The figure shows three views and two pictorial views of one solid part (mm, origin at its lowest corner). Answer the questions. Coordinates: 2 decimals unless noted, no trailing zeros. Order: outer loops, then holes, each group sorted by start corner. A loop starts at its lowest first (then second) coordinate and runs counter-clockwise, first axis right, second up. Notation, with made-up numbers: M 55.25,71 L 76.25,71 A7 cw 76.25,82 Z; hole C -36,64.5 d6. An arc over 180 degrees is marked long. Answer in a Markdown table with one row per item. Add a question column.
Item 1: The mould has two halves that part along X. Classify the marked faces 1, 2 and 3: released by +X, released by -X, zero draft, split by the parting line, or undercut.
Item 2: The part is cut by section C-C (z = 33.5). Write down the section's boundary in (x, y).
Item 3: The part is cut by section A-A (y = 2). State how many separate pieces and enclosed holes the cut face has.
Item 4: Flat-ended cylindrical pins translate along their axes: pin 1 Ø3 at (x, z) = (10.38, 29.63) entering from -Y; pin 2 Ø2 at (y, z) = (2, 22) entering from -X; pin 3 Ø1.7 at (x, z) = (2.69, 18.73) entering from +Y. Find the tip coordinate at first contact, or state that the pin passes through.
Item 5: Consider line 1 (X direction, y = 2, z = 18) (1 decimal); line 2 (X direction, y = 0.5, z = 18.5) (1 decimal); line 3 (X direction, y = 4.25, z = 11) (1 decimal). Determine where each line is inside the solid, lowest interval first. Write a range as from..to.
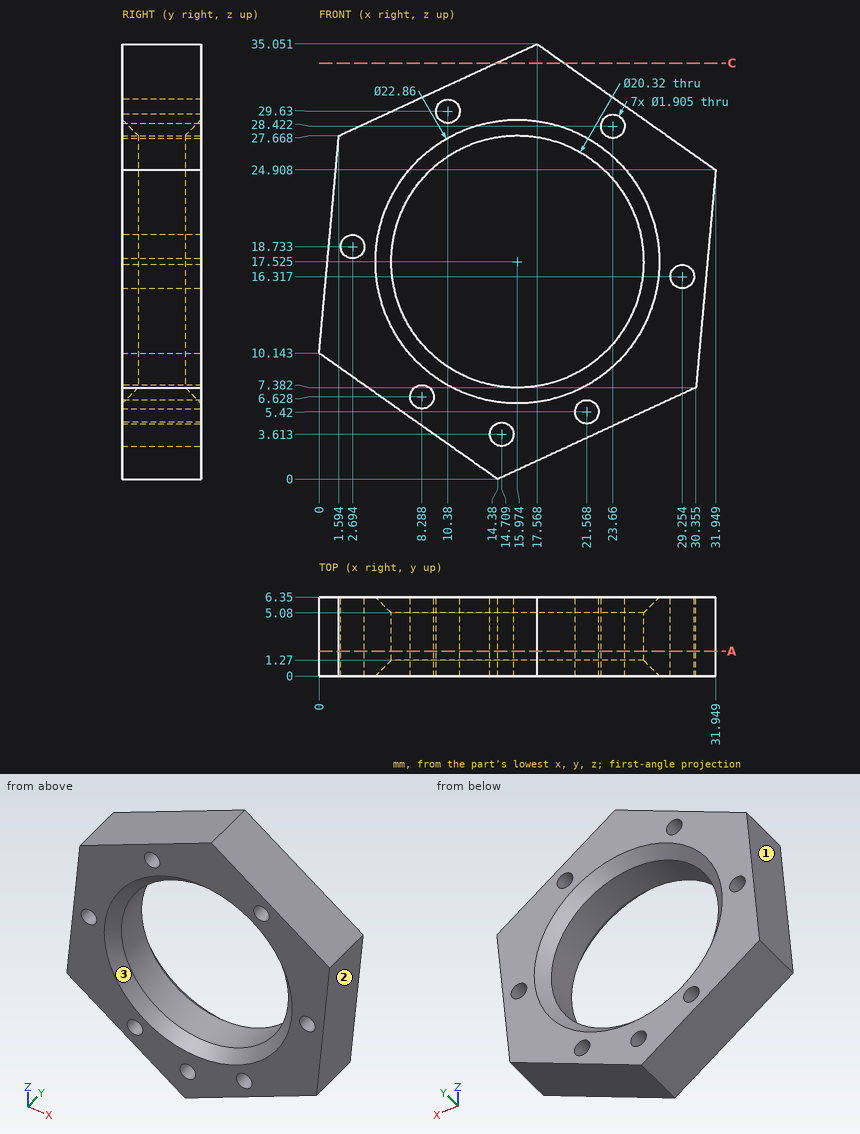
Reply:
| question | item | result |
|---|---|---|
| 1 | face 1 | released by -X |
| 1 | face 2 | released by +X |
| 1 | face 3 | undercut |
| 2 | outline | M 14.21,0 L 19.77,0 L 19.77,6.35 L 14.21,6.35 Z |
| 3 | separate pieces | 1 |
| 3 | enclosed holes | 8 |
| 4 | pin 1 | stops at y = 0 |
| 4 | pin 2 | stops at x = 0.99 |
| 4 | pin 3 | passes through |
| 5 | line 1 | x = 0.7..2.1, 3.3..5.8, 26.1..31.3 |
| 5 | line 2 | x = 0.8..1.8, 3.6..5.1, 26.9..31.4 |
| 5 | line 3 | x = 0.1..8.2, 23.8..30.7 |
